```python
from build123d import *

# Parameters (mm, degrees)
SKETCH1_R           = 1.75
BOSS_EXTRUDE1_DEPTH = 5
SKETCH2_W           = 35
SKETCH2_H           = 20
SKETCH2_W_2         = 22.6
SKETCH2_H_2         = 12
BOSS_EXTRUDE2_DEPTH = 3
SKETCH3_W           = 15.4
SKETCH3_H           = 20
CUT_EXTRUDE1_DEPTH  = 76.166481892
SKETCH4_R           = 1
CUT_EXTRUDE2_DEPTH  = 7
SKETCH5_W           = 38
SKETCH5_H           = 25
BOSS_EXTRUDE3_DEPTH = 5
SKETCH6_R           = 2.3
CUT_EXTRUDE3_DEPTH  = 4
FILLET1_R           = 4
SKETCH2_2_W         = 22.6
SKETCH2_2_H         = 12
CUT_EXTRUDE4_DEPTH  = 1
CUT_EXTRUDE5_DEPTH  = 65.832264344
CUT_EXTRUDE6_DEPTH  = 65.627567647
SKETCH9_W           = 38
SKETCH9_H           = 4.5
CUT_EXTRUDE7_DEPTH  = 4


with BuildPart() as part:
    # Sketch1 → Boss-Extrude1 (new body)
    with BuildSketch(Plane(origin=(0, 0, 0), x_dir=(1, 0, 0), z_dir=(0, 1, 0))):
        Polygon((0, 15), (0, 33.819660113), (10, 45), (26, 45), (36, 35), (60, 35), (60, 15), (36, 15), (26, 0), (10, 0), align=None)
        with Locations(Location((5, 25, 0), (0, 0, 270))):
            Circle(SKETCH1_R, mode=Mode.SUBTRACT)
        with Locations(Location((13, 5, 0), (0, 0, 270))):
            Circle(SKETCH1_R, mode=Mode.SUBTRACT)
        with Locations(Location((23, 5, 0), (0, 0, 270))):
            Circle(SKETCH1_R, mode=Mode.SUBTRACT)
    extrude(amount=BOSS_EXTRUDE1_DEPTH)

    # Sketch2 → Boss-Extrude2 (add)
    with BuildSketch(Plane.XZ):
        with Locations((27.1, -25)):
            Rectangle(SKETCH2_W, SKETCH2_H)
        with Locations((27.1, -25)):
            Rectangle(SKETCH2_W_2, SKETCH2_H_2, mode=Mode.SUBTRACT)
    extrude(amount=BOSS_EXTRUDE2_DEPTH)

    # Sketch3 → Cut-Extrude1 (cut, through all)
    with BuildSketch(Plane.XZ):
        with Locations((52.3, -25)):
            Rectangle(SKETCH3_W, SKETCH3_H)
    extrude(amount=-CUT_EXTRUDE1_DEPTH, mode=Mode.SUBTRACT)

    # Sketch4 → Cut-Extrude2 (cut)
    with BuildSketch(Plane.XZ.offset(3)):
        with Locations(Location((13.52, -25, 0), (0, 0, 270))):
            Circle(SKETCH4_R)
        with Locations(Location((40.67, -25, 0), (0, 0, 270))):
            Circle(SKETCH4_R)
    extrude(amount=-CUT_EXTRUDE2_DEPTH, mode=Mode.SUBTRACT)

    # Sketch5 → Boss-Extrude3 (add)
    with BuildSketch(Plane(origin=(0, 0, -35), x_dir=(-1, 0, 0), z_dir=(0, 0, -1))):
        with Locations((-21.4, -0.25)):
            Rectangle(SKETCH5_W, SKETCH5_H)
    extrude(amount=BOSS_EXTRUDE3_DEPTH)

    # Sketch6 → Cut-Extrude3 (cut)
    with BuildSketch(Plane(origin=(0, 0, -40), x_dir=(-1, 0, 0), z_dir=(0, 0, -1))):
        with Locations((-21.39853967, -0.25)):
            Circle(SKETCH6_R)
    extrude(amount=-CUT_EXTRUDE3_DEPTH, mode=Mode.SUBTRACT)

    # Fillet1
    fillet1_edges = [part.edges().sort_by_distance(p)[0] for p in [
        (2.4, -12.75, -37.5),
        (40.4, 12.25, -37.5),
        (40.4, -12.75, -37.5),
        (2.4, 12.25, -37.5),
        (44.6, 1, -35),
        (44.6, 1, -15),
    ]]
    fillet(fillet1_edges, radius=FILLET1_R)

    # Sketch2_2 → Cut-Extrude4 (cut)
    with BuildSketch(Plane.XZ):
        with Locations((27.1, -25)):
            Rectangle(SKETCH2_2_W, SKETCH2_2_H)
    extrude(amount=-CUT_EXTRUDE4_DEPTH, mode=Mode.SUBTRACT)

    # Sketch7 → Cut-Extrude5 (cut, through all)
    with BuildSketch(Plane.XZ.offset(-1)):
        with BuildLine():
            Line((26.1, -22.5), (26.945643943, -22.5))
            ThreePointArc((26.945643943, -22.5), (38.4, -25), (26.945643943, -27.5))
            Line((26.945643943, -27.5), (26.1, -27.5))
            ThreePointArc((26.1, -27.5), (23.6, -25), (26.1, -22.5))
        make_face()
    extrude(amount=-CUT_EXTRUDE5_DEPTH, mode=Mode.SUBTRACT)

    # Sketch8 → Cut-Extrude6 (cut, through all)
    with BuildSketch(Plane.XZ):
        Polygon((26, -45), (31, -40), (23.684912343, -40), (19.112166997, -40), (5.527864045, -40), (10, -45), align=None)
    extrude(amount=-CUT_EXTRUDE6_DEPTH, mode=Mode.SUBTRACT)

    # Sketch9 → Cut-Extrude7 (cut)
    with BuildSketch(Plane.XY.offset(-35)):
        with Locations((21.4, 7.25)):
            Rectangle(SKETCH9_W, SKETCH9_H)
    extrude(amount=-CUT_EXTRUDE7_DEPTH, mode=Mode.SUBTRACT)


solid = part.part
```
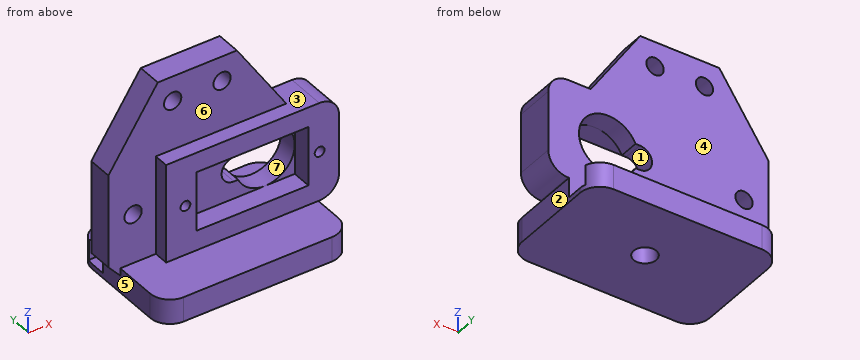
Here's how the part is built. I have some questions about the finished solid (model axes, mm). Face numbers are marked on the shaded views. A direction names the side the tool comes from. Round coordinates to 2 decimals unless told otherwise and drop trailing zeros. Write each loop counter-clockwise with the first axis right and the second up, starting at its lowest first coordinate (ties: lowest second). Pieces come first, ordered by that corner, then holes.
Q1. If we section it at A-A on z = -21.5: Write out the boundary of the cut face in (x, y), plus the area to 3 significant figures.
Q2. Please list where these lines run through material, in increasing order: probe 1 along X at (y, z) = (1.75, -25); probe 2 along Y at (x, z) = (10, -37.5); probe 3 along X at (y, z) = (1.55, -5).
Q3. If we section it at B-B on x = 30: Write out the boundary of the cut face in (y, z).
Q4. Which directions (+Z, -Z, +X, -X, +Y, -Y) give clear straight access to the entire face, cutting with the end or side of a thin tool? Please do the marked faces 1, 2, 3 and 4.
Q5. If we mould it in two halves opening along X, with no side actions, what happens to the marked faces 5, 6 and 7? For each: +X half, -X half, draft (parallel to the pull), parting line (faces both ways), or undercut.
Q6. If we section it at D-D on x = 13.52: Write out the boundary of the cut face in (y, z).
Q7. Will these pins go through, and if not, where does the flat tip stop? P1, Ø1, axis at x = 17.5, z = -27.5, coming from the -Y side; P2, Ø5, axis at x = 30, z = -25.5, coming from the -Y side; P3, Ø10, axis at y = -8, z = -31, coming from the -X side; P4, Ø4.5, axis at x = 13, z = -5, coming from the -Y side.
Q8. If we section it at C-C on x = 7.5: Write out the boundary of the cut face in (y, z).
Answer below:
1. outline: (0, 0) - (9.6, 0) - (9.6, -3) - (15.8, -3) - (15.8, 1) - (27.53, 1) - (27.53, 5) - (0, 5) - close; (37.27, 1) - (38.4, 1) - (38.4, -3) - (44.6, -3) - (44.6, 5) - (37.27, 5) - close
1. area: 199 mm2
2. probe 1: x = 0 to 3.25, 6.75 to 12.52, 14.52 to 23.6, 38.4 to 39.67, 41.67 to 44.6
2. probe 2: y = -12.75 to 5, 9.5 to 12.25
2. probe 3: x = 6.67 to 11.25, 14.75 to 21.25, 24.75 to 29.33
3. outline: (-12.75, -40) - (12.25, -40) - (12.25, -35) - (9.5, -35) - (9.5, -39) - (5, -39) - (5, -30.5) - (1, -30.5) - (1, -31) - (-3, -31) - (-3, -35) - (-12.75, -35) - close; (-3, -19) - (1, -19) - (1, -19.5) - (5, -19.5) - (5, -6) - (0, -6) - (0, -15) - (-3, -15) - close
4. face 1: +Y, -Y
4. face 2: -Z, +X, +Y, -Y
4. face 3: +Z, +X, -Y
4. face 4: +Z, +X, -X
5. face 5: -X half
5. face 6: draft
5. face 7: undercut
6. outline: (-12.75, -40) - (12.25, -40) - (12.25, -35) - (9.5, -35) - (9.5, -39) - (5, -39) - (5, -6.67) - (0, -6.67) - (0, -15) - (-3, -15) - (-3, -24) - (4, -24) - (4, -26) - (-3, -26) - (-3, -35) - (-12.75, -35) - close; (0, -3.33) - (5, -3.33) - (5, 0) - (0, 0) - close
7. P1: stops at y = 1
7. P2: passes through
7. P3: stops at x = 2.4
7. P4: stops at y = 0
8. outline: (-12.75, -40) - (12.25, -40) - (12.25, -35) - (9.5, -35) - (9.5, -39) - (5, -39) - (5, -3.75) - (0, -3.75) - (0, -35) - (-12.75, -35) - close
